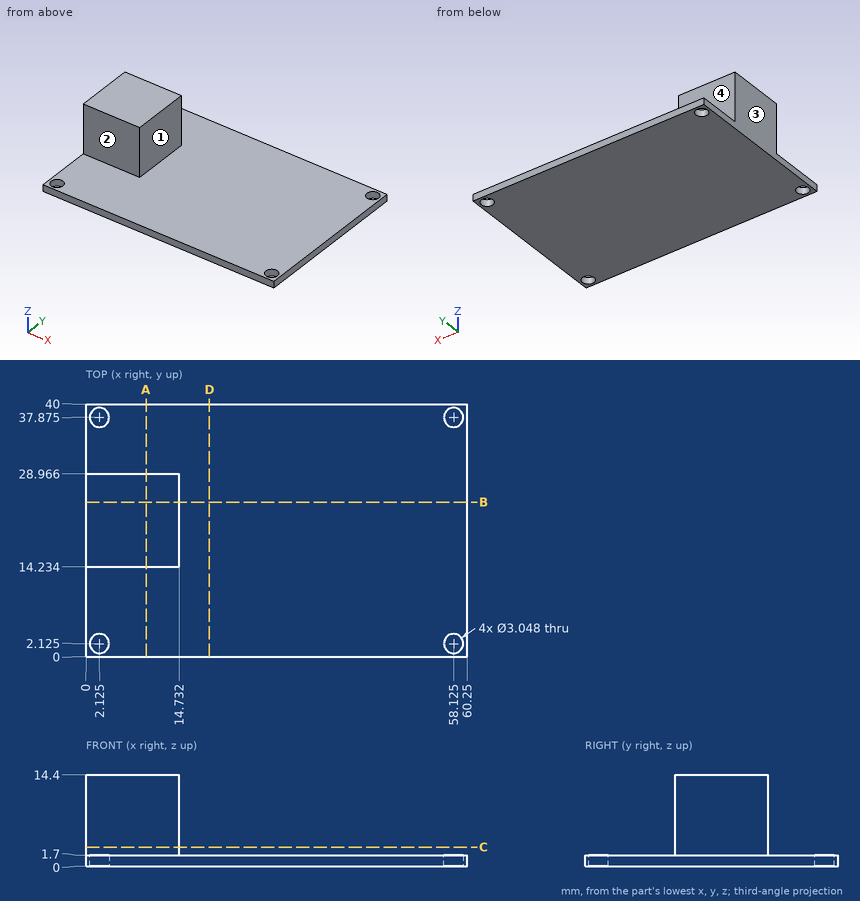
Geometry: see drawing. Coordinates: mm, zero at the bounding-box minimum. A direction names the side the tool comes from. Round coordinates to 2 decimals unless told otherwise and drop trailing zeros. Loops run counter-clockwise (first coordinate to the right, second up) from the corner with the lowest first, then second, coordinate; pieces in that order, holes last. Notation, with made-up numbers: M -9.5,24 L 7.5,24 A27 cw 7.5,52 Z; hole C 70,-3 d6. An arc over 180 degrees is marked long. Use a Markdown table: item, result. Add a question column.
1. Ray query, line 1 along Z through (x, y) = (19, 22.5); line 2 along Y through (x, z) = (13, 11.25); line 3 along X through (y, z) = (22, 4). Return the intervals inside material, ascending. Write a range as [from, to].
2. Cut plane A-A, the plane x = 9.5. Output: boundary loops of the cut face in (y, z), and give its area (3 significant figures).
3. Set-up query: the marked faces 1, 2, 3 and 4. Return all of +Z, -Z, +X, -X, +Y, -Y with unobstructed straight access to the full face (end or side cutting, diameter ignored); none if empty.
4. Cut plane C-C, the plane z = 3. Output: boundary loops of the cut face in (x, y), and give its area (3 significant figures).
5. Cut plane B-B, the plane y = 24.5. Output: boundary loops of the cut face in (x, z).
6. Contact query for flat-ended pins moving along their axis: pin 1 (1.5 mm diameter, centred on x = 19.5, y = 34.5, fed in from +Z); pin 2 (6 mm diameter, centred on x = 7.5, z = 7.5, fed in from -Y). Output: stop coordinate, or through.
7. Cut plane D-D, the plane x = 19.5. Output: boundary loops of the cut face in (y, z), and give its area (3 significant figures).
Solution:
| question | item | result |
|---|---|---|
| 1 | line 1 | z = [0, 1.7] |
| 1 | line 2 | y = [14.23, 28.97] |
| 1 | line 3 | x = [0, 14.73] |
| 2 | outline | M 0,0 L 40,0 L 40,1.7 L 28.97,1.7 L 28.97,14.4 L 14.23,14.4 L 14.23,1.7 L 0,1.7 Z |
| 2 | area | 255 mm2 |
| 3 | face 1 | +Z, +X, +Y, -Y |
| 3 | face 2 | +Z, +X, -X, -Y |
| 3 | face 3 | +Z, -Z, -X, +Y, -Y |
| 3 | face 4 | +Z, +X, -X, +Y |
| 4 | outline | M 0,14.23 L 14.73,14.23 L 14.73,28.97 L 0,28.97 Z |
| 4 | area | 217 mm2 |
| 5 | outline | M 0,0 L 60.25,0 L 60.25,1.7 L 14.73,1.7 L 14.73,14.4 L 0,14.4 Z |
| 6 | pin 1 | stops at z = 1.7 |
| 6 | pin 2 | stops at y = 14.23 |
| 7 | outline | M 0,0 L 40,0 L 40,1.7 L 0,1.7 Z |
| 7 | area | 68.0 mm2 |
